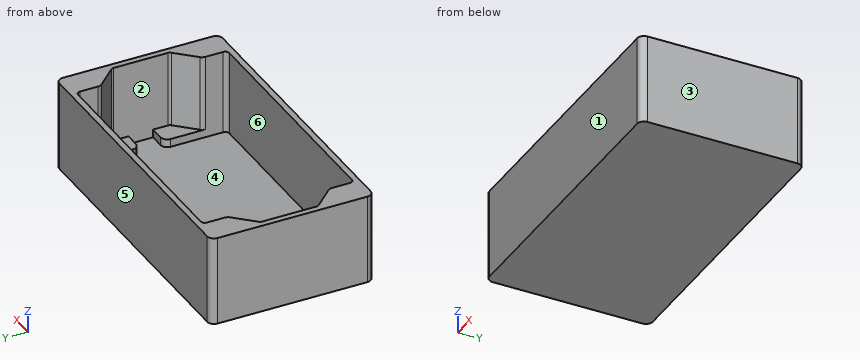
from build123d import *

# Parameters (mm, degrees)
SKETCH1_W           = 220
SKETCH1_H           = 120
BOSS_EXTRUDE1_DEPTH = 33
CUT_EXTRUDE1_DEPTH  = 56
CUT_EXTRUDE2_DEPTH  = 6
FILLET1_R           = 5


with BuildPart() as part:
    # Sketch1 → Boss-Extrude1 (new, symmetric)
    with BuildSketch(Plane.XY):
        Rectangle(SKETCH1_W, SKETCH1_H)
    extrude(amount=BOSS_EXTRUDE1_DEPTH, both=True)

    # Sketch2 → Cut-Extrude1 (cut)
    with BuildSketch(Plane.XY.offset(33)):
        with BuildLine():
            Line((-87, 55.5), (87, 55.5))
            ThreePointArc((87, 55.5), (89.121320344, 54.621320344), (90, 52.5))
            Line((90, 52.5), (90, 39.49693341))
            ThreePointArc((90, 39.49693341), (90.356635174, 37.642435339), (91.375665238, 36.052488965))
            Line((91.375665238, 36.052488965), (104.674600857, 22.059000191))
            ThreePointArc((104.674600857, 22.059000191), (105.286018895, 21.105032366), (105.5, 19.992333524))
            Line((105.5, 19.992333524), (105.5, -19.992333524))
            ThreePointArc((105.5, -19.992333524), (105.286018895, -21.105032366), (104.674600857, -22.059000191))
            Line((104.674600857, -22.059000191), (91.375665238, -36.052488965))
            ThreePointArc((91.375665238, -36.052488965), (90.356635174, -37.642435339), (90, -39.49693341))
            Line((90, -39.49693341), (90, -52.5))
            ThreePointArc((90, -52.5), (89.121320344, -54.621320344), (87, -55.5))
            Line((87, -55.5), (-87, -55.5))
            ThreePointArc((-87, -55.5), (-89.121320344, -54.621320344), (-90, -52.5))
            Line((-90, -52.5), (-90, -39.49693341))
            ThreePointArc((-90, -39.49693341), (-90.356635174, -37.642435339), (-91.375665238, -36.052488965))
            Line((-91.375665238, -36.052488965), (-104.674600857, -22.059000191))
            ThreePointArc((-104.674600857, -22.059000191), (-105.286018895, -21.105032366), (-105.5, -19.992333524))
            Line((-105.5, -19.992333524), (-105.5, 19.992333524))
            ThreePointArc((-105.5, 19.992333524), (-105.286018895, 21.105032366), (-104.674600857, 22.059000191))
            Line((-104.674600857, 22.059000191), (-91.375665238, 36.052488965))
            ThreePointArc((-91.375665238, 36.052488965), (-90.356635174, 37.642435339), (-90, 39.49693341))
            Line((-90, 39.49693341), (-90, 52.5))
            ThreePointArc((-90, 52.5), (-89.121320344, 54.621320344), (-87, 55.5))
        make_face()
    extrude(amount=-CUT_EXTRUDE1_DEPTH, mode=Mode.SUBTRACT)

    # Sketch3 → Cut-Extrude2 (cut)
    with BuildSketch(Plane.XY.offset(-23)):
        with BuildLine():
            Line((-90, 52.5), (-90, 39.49693341))
            Line((-90, 39.49693341), (-90, 14))
            ThreePointArc((-90, 14), (-91.464466094, 10.464466094), (-95, 9))
            Line((-95, 9), (-105.5, 9))
            Line((-105.5, 9), (-105.5, -9))
            Line((-105.5, -9), (-95, -9))
            ThreePointArc((-95, -9), (-91.464466094, -10.464466094), (-90, -14))
            Line((-90, -14), (-90, -39.49693341))
            Line((-90, -39.49693341), (-90, -52.5))
            ThreePointArc((-90, -52.5), (-89.121320344, -54.621320344), (-87, -55.5))
            Line((-87, -55.5), (87, -55.5))
            ThreePointArc((87, -55.5), (89.121320344, -54.621320344), (90, -52.5))
            Line((90, -52.5), (90, -39.49693341))
            Line((90, -39.49693341), (90, -14))
            ThreePointArc((90, -14), (91.464466094, -10.464466094), (95, -9))
            Line((95, -9), (105.5, -9))
            Line((105.5, -9), (105.5, 9))
            Line((105.5, 9), (95, 9))
            ThreePointArc((95, 9), (91.464466094, 10.464466094), (90, 14))
            Line((90, 14), (90, 39.49693341))
            Line((90, 39.49693341), (90, 52.5))
            ThreePointArc((90, 52.5), (89.121320344, 54.621320344), (87, 55.5))
            Line((87, 55.5), (-87, 55.5))
            ThreePointArc((-87, 55.5), (-89.121320344, 54.621320344), (-90, 52.5))
        make_face()
    extrude(amount=-CUT_EXTRUDE2_DEPTH, mode=Mode.SUBTRACT)

    # Fillet1
    fillet1_edges = [part.edges().sort_by_distance(p)[0] for p in [
        (-110, 60, 0),
        (110, 60, 0),
        (110, -60, 0),
        (-110, -60, 0),
    ]]
    fillet(fillet1_edges, radius=FILLET1_R)


solid = part.part
Input: part model. Units: mm. Frame: model coordinates. Face numbers are marked on the shaded views. A direction names the side the tool comes from. Give positions to 0.01 mm unless a question says otherwise; leave off trailing zeros. Order: outer loops, then holes, each group sorted by start corner. A loop starts at its lowest first (then second) coordinate and runs counter-clockwise, first axis right, second up. Notation, with made-up numbers: M -18.75,5.5 L -12.75,5.5 A25 cw -12.75,43.5 Z; hole C 33.5,30.25 d5. An arc over 180 degrees is marked long. Answer as a JSON object with one key per item and string values.
1. Pull-direction query (X, two-part tool) for the marked faces 1, 2, 3 and 4; classes: +X half, -X half, draft (parallel to the pull), parting line (faces both ways), or undercut.
Result sheet:
{"face 1": "draft", "face 2": "undercut", "face 3": "+X half", "face 4": "undercut"}
2. Cut plane D-D, the plane y = 31.5. Output: boundary loops of the cut face in (x, z), and give its area (3 significant figures).
Result sheet:
{"outline": "M -110,-33 L 110,-33 L 110,33 L 95.7,33 L 95.7,-23 L 90,-23 L 90,-29 L -90,-29 L -90,-23 L -95.7,-23 L -95.7,33 L -110,33 Z", "area": "2,720 mm²"}
3. Ray query, line 1 (Y direction, x = -31, z = 4.5); line 2 (X direction, y = 12.5, z = -3.5); line 3 (X direction, y = 50, z = 26). Return the intervals inside material, ascending. Write a range as [from, to].
Result sheet:
{"line 1": "[-60, -55.5], [55.5, 60]", "line 2": "[-110, -105.5], [105.5, 110]", "line 3": "[-110, -90], [90, 110]"}
4. First-contact query: P1, Ø8, axis at x = -63, y = -45.5, coming from the +Z side. Flat tip, straight axial feed; report the tip coordinate or a pass-through.
Result sheet:
{"P1": "z = -29"}
5. Cut plane C-C, the plane x = 69.5. Output: boundary loops of the cut face in (y, z), and give its area (3 significant figures).
Result sheet:
{"outline": "M -60,-33 L 60,-33 L 60,33 L 55.5,33 L 55.5,-29 L -55.5,-29 L -55.5,33 L -60,33 Z", "area": "1,040 mm²"}
6. Reachability of the marked faces 5 and 6 from +Z, -Z, +X, -X, +Y, -Y: full face, straight path, thin tool, end or side. Return the list, or none.
Result sheet:
{"face 5": "+Z, -Z, +X, -X, +Y", "face 6": "+Z"}
7. Cut plane B-B, the plane y = 6. Output: boundary loops of the cut face in (x, z), and give its area (3 significant figures).
Result sheet:
{"outline": "M -110,-33 L 110,-33 L 110,33 L 105.5,33 L 105.5,-29 L -105.5,-29 L -105.5,33 L -110,33 Z", "area": "1,440 mm²"}
